from build123d import *

# Parameters (mm, degrees)
BOSS_EXTRUDE1_DEPTH             = 20
M3X0_5_TAPPED_HOLE1_D           = 2.5
M3X0_5_TAPPED_HOLE1_CSINK_D     = 3.05
M3X0_5_TAPPED_HOLE1_CSINK_ANGLE = 90
CHAMFER1_SIZE                   = 2.5
CHAMFER1_SIZE2                  = 4.330127019


with BuildPart() as part:
    # Sketch1 → Boss-Extrude1 (new body)
    with BuildSketch(Plane.XY):
        Polygon((0, 0), (4, 0), (4, -3.637956731), (10, -3.637956731), (10, -6.68821772), (-3, -6.68821772), (-3, 5.414430721), (3, 5.414430721), (3, 1.7), (0, 1.7), align=None)
    extrude(amount=BOSS_EXTRUDE1_DEPTH)

    # M3x0.5 Tapped Hole1 (through all)
    with Locations(Plane(origin=(0, -3.637956731, 0), x_dir=(1, 0, 0), z_dir=(0, 1, 0))):
        with Locations((7.5, -10)):
            CounterSinkHole(M3X0_5_TAPPED_HOLE1_D / 2, M3X0_5_TAPPED_HOLE1_CSINK_D / 2, counter_sink_angle=M3X0_5_TAPPED_HOLE1_CSINK_ANGLE)

    # Chamfer1
    chamfer1_edges = [part.edges().sort_by_distance(p)[0] for p in [
        (3, 5.414430721, 10),
    ]]
    chamfer1_side = [part.faces().sort_by_distance(p)[0] for p in [
        (3, 3.55721536, 10),
    ]]
    chamfer(chamfer1_edges, length=CHAMFER1_SIZE, length2=CHAMFER1_SIZE2, reference=chamfer1_side[0])


solid = part.part
For this review, take the finished solid that the model builds, in its own axes (mm). A direction names the side the tool comes from. Round coordinates to 2 decimals unless told otherwise and drop trailing zeros. Loops run counter-clockwise (first coordinate to the right, second up) from the corner with the lowest first, then second, coordinate; pieces in that order, holes last. Notation, with made-up numbers: (-19, 78.25) - (24, 78.25) arc R20 ccw to (24, 90.25) - close; hole circle Ø3 at (-31.5, 0.5). An arc over 180 degrees is marked (long way). One line per item, written item: value. Start each with the question number.
Item 1: The part is to be moulded in two halves that separate along Z. For faces 4 (the cylindrical face through (8.421, -5.32, 9.155)), 5 (the flat face through (5.6, -3.638, 9.9)), 6 (the flat face through (2, -2, 20)), 7 (the flat face through (2, -2, 0)), say which applies: +Z half, -Z half, draft (parallel to the pull), parting line (faces both ways), or undercut.
Item 2: For L1, parallel to X at y = -5.3, z = 10; L2, parallel to Z at x = 7.5, y = -5.8; L3, parallel to Y at x = 5, z = 9.5, list the stretches that pass through material, from the lowest coordinate up.
Item 3: Take a section at B-B (z = 10). Give the boundary of the cut face in (x, y) (3 decimals).
Item 4: Clearance check with flat-ended pins moving along their axes: pin 1 Ø1 at (y, z) = (2.5, 7) entering from +X; pin 2 Ø3 at (x, z) = (7.5, 10) entering from +Y; pin 3 Ø1.5 at (x, y) = (4.5, -3.5) entering from -Z; pin 4 Ø1.8 at (x, z) = (6, 10.5) entering from +Y. State where each tip first meets the part, or that it passes through.
Item 5: Take a section at A-A (x = 7.5). Give the boundary of the cut face in (y, z) (3 decimals).
Item 6: Take a section at C-C (z = 12). Give the boundary of the cut face in (x, y).
Item 7: For faces 1 (the flat face through (4, -6.688, 10)), 2 (the flat face through (4, -2, 10)), 3 (the flat face through (2, 1.7, 10)), list the 3-axis set-ups (+Z, -Z, +X, -X, +Y, -Y) from which the entire face can be reached by the end or side of a thin tool; tool diameter is ignored.
Item 8: Take a section at D-D (y = -1.25). Give the boundary of the cut face in (x, z).
Answer below:
1. face 4: undercut
1. face 5: draft
1. face 6: +Z half
1. face 7: -Z half
2. L1: x = -3 to 6.25, 8.75 to 10
2. L2: z = 0 to 8.75, 11.25 to 20
2. L3: y = -6.69 to -3.64
3. outline: (-3, -6.688) - (6.25, -6.688) - (6.25, -3.913) - (5.975, -3.638) - (4, -3.638) - (4, 0) - (0, 0) - (0, 1.7) - (3, 1.7) - (3, 2.914) - (-1.33, 5.414) - (-3, 5.414) - close; (8.75, -6.688) - (10, -6.688) - (10, -3.638) - (9.025, -3.638) - (8.75, -3.913) - close
4. pin 1: stops at x = 3
4. pin 2: stops at y = -3.66
4. pin 3: stops at z = 0
4. pin 4: stops at y = -3.64
5. outline: (-6.688, 0) - (-3.638, 0) - (-3.638, 8.475) - (-3.913, 8.75) - (-6.688, 8.75) - close; (-6.688, 11.25) - (-3.913, 11.25) - (-3.638, 11.525) - (-3.638, 20) - (-6.688, 20) - close
6. outline: (-3, -6.69) - (10, -6.69) - (10, -3.64) - (4, -3.64) - (4, 0) - (0, 0) - (0, 1.7) - (3, 1.7) - (3, 2.91) - (-1.33, 5.41) - (-3, 5.41) - close
7. face 1: +Z, -Z, +X, -X, -Y
7. face 2: +Z, -Z, +X, +Y
7. face 3: +Z, -Z, +X
8. outline: (-3, 0) - (4, 0) - (4, 20) - (-3, 20) - close
